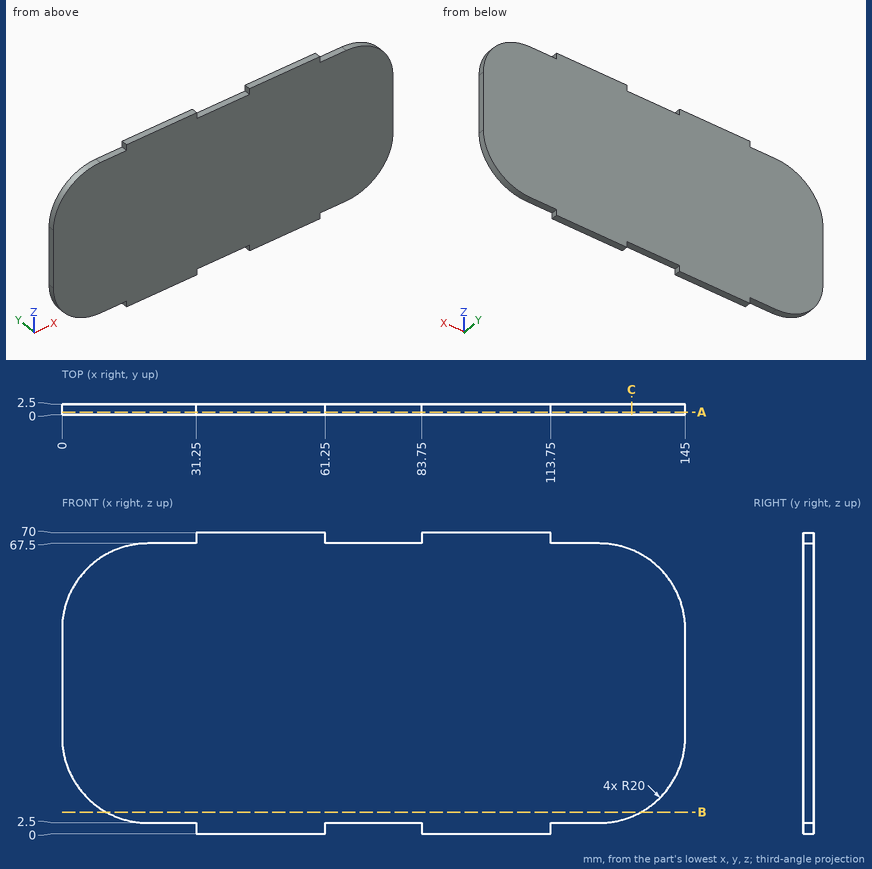
Answer from the drawing. Dimensions are ordinates in mm from the lowest x, y and z of the part. Give positions to 0.01 mm unless a question says otherwise; leave off trailing zeros. Loops run counter-clockwise (first coordinate to the right, second up) from the corner with the lowest first, then second, coordinate; pieces in that order, holes last.
Item 1: A cutting plane is placed at C-C (x = 132.5). Give the vertices of the cut face in (y, z), then the cut area to 3 significant figures.
Derived:
outline: (0, 3.96) - (2.5, 3.96) - (2.5, 66.04) - (0, 66.04) - close
area: 155 mm2
Item 2: Each of these flat-tipped pins is pushed along its axis until it touches: pin 1 Ø1.2 at (x, y) = (26.5, 2) entering from +Z; pin 2 Ø1.5 at (y, z) = (0.5, 12.5) entering from -X; pin 3 Ø1.2 at (y, z) = (2, 68.5) entering from +X. Where does it stop, or does it pass through?
Derived:
pin 1: stops at z = 67.5
pin 2: stops at x = 2.27
pin 3: stops at x = 113.75
Item 3: Find the intervals of material crossed by line 1 along Z through (x, y) = (30, 1.3); line 2 along X through (y, z) = (0.9, 51.5); line 3 along X through (y, z) = (1.25, 9), in increasing order.
Derived:
line 1: z = 2.5 to 67.5
line 2: x = 0.4 to 144.6
line 3: x = 5.24 to 139.76
Item 4: A cutting plane is placed at B-B (z = 5). Give the vertices of the cut face in (x, y).
Derived:
outline: (10.32, 0) - (134.68, 0) - (134.68, 2.5) - (10.32, 2.5) - close
Item 5: A cutting plane is placed at A-A (y = 0.6). Give the vertices of the cut face in (x, z), then the cut area to 3 significant figures.
Derived:
outline: (0, 22.5) arc R20 ccw to (20, 2.5) - (31.25, 2.5) - (31.25, 0) - (61.25, 0) - (61.25, 2.5) - (83.75, 2.5) - (83.75, 0) - (113.75, 0) - (113.75, 2.5) - (125, 2.5) arc R20 ccw to (145, 22.5) - (145, 47.5) arc R20 ccw to (125, 67.5) - (113.75, 67.5) - (113.75, 70) - (83.75, 70) - (83.75, 67.5) - (61.25, 67.5) - (61.25, 70) - (31.25, 70) - (31.25, 67.5) - (20, 67.5) arc R20 ccw to (0, 47.5) - close
area: 9,380 mm2
